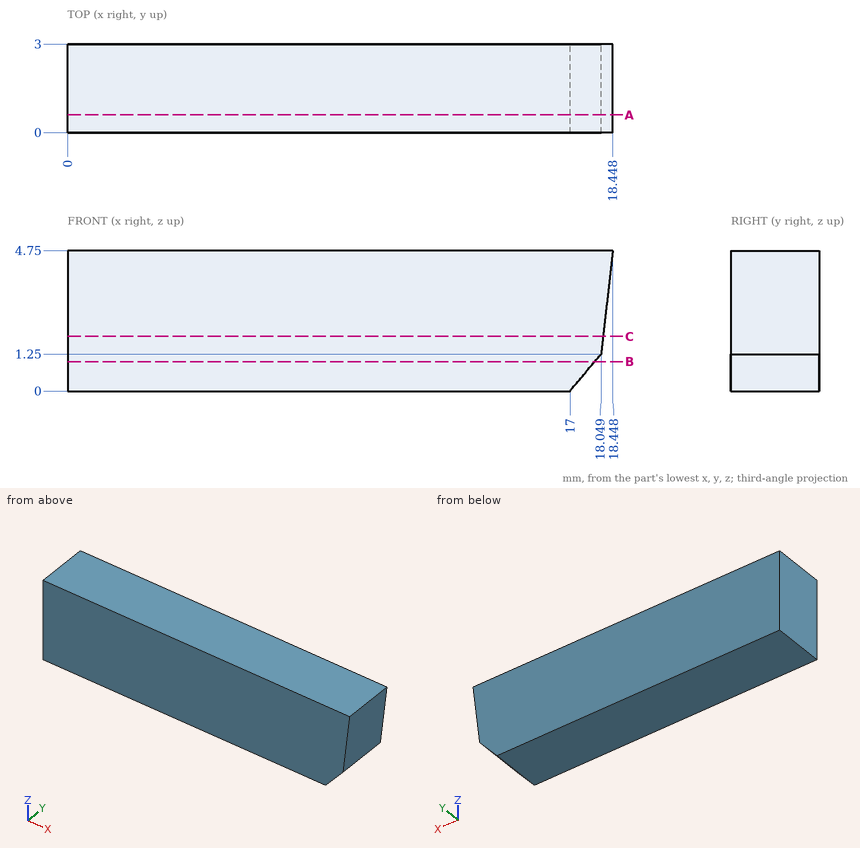
Could you check a few things on this drawing? It's one solid part, dimensions in mm from its lowest x, y, z. Give positions to 0.01 mm unless a question says otherwise; leave off trailing zeros. Write each loop counter-clockwise with the first axis right and the second up, starting at its lowest first coordinate (ties: lowest second). Pieces come first, ordered by that corner, then holes. Notation, with made-up numbers: (49.5, -2.75) -> (100.5, -2.75) arc R26 cw to (100.5, 31.25) -> close; hole circle Ø6 at (58, 79). An arc over 180 degrees is marked (long way). Answer as CSV lines item,"result". Start each with the question number.
(1) If we section it at A-A, the plane y = 0.6: Write out the boundary of the cut face in (x, z).
(2) Please list where these lines run through material, in increasing order: line 1 (X direction, y = 2.25, z = 2.7); line 2 (X direction, y = 1.25, z = 3.85) (1 decimal).
(3) If we section it at B-B, the plane z = 1: Write out the boundary of the cut face in (x, y), and give its area (3 significant figures).
(4) If we section it at C-C, the plane z = 1.85: Write out the boundary of the cut face in (x, y).
Answer list:
1,outline,"(0, 0) -> (17, 0) -> (18.05, 1.25) -> (18.45, 4.75) -> (0, 4.75) -> close"
2,line 1,"0 to 18.21"
2,line 2,"0 to 18.3"
3,outline,"(0, 0) -> (17.84, 0) -> (17.84, 3) -> (0, 3) -> close"
3,area,"53.5 mm^2"
4,outline,"(0, 0) -> (18.12, 0) -> (18.12, 3) -> (0, 3) -> close"
